Part model, mm, in its own coordinate system. A direction names the side the tool comes from. Coordinates: 2 decimals unless noted, no trailing zeros. Order: outer loops, then holes, each group sorted by start corner. A loop starts at its lowest first (then second) coordinate and runs counter-clockwise, first axis right, second up. Notation, with made-up numbers: (1.5, 36) - (10.5, 36) arc R20 ccw to (10.5, 62) - close; hole circle Ø8 at (28, 52). An arc over 180 degrees is marked (long way). Use a Markdown table: item, result. Add a question column.
1) Two-plate mould, pull along Y, no slides. Class faces 3 (the face through (1, -18, -45)), 4 (the face through (1.5, -15.9, -6.3)), 5 (the face through (1, -15, -30)): +Y half, -Y half, draft (parallel to the pull), parting line (faces both ways), or undercut.
2) Tool access for faces 1 (the face through (1, -18, -15)), 2 (the face through (1.5, -15.9, -51.3)): list every direction of +Z, -Z, +X, -X, +Y, -Y with a clear straight run to the whole face (end or side of a thin tool).
3) Wall check: L1, parallel to Y at x = 0.7, z = -7.5; L2, parallel to Y at x = 2.2, z = -17.5; L3, parallel to Z at x = 0.7, y = -18.5. Give the ranges that are in metal, low to high. Write a range as [from, to].
4) Saw through at B-B on y = -8.25. List the corners of the cut face in (x, z), then the cut area to 3 significant figures.
5) Saw through at D-D on z = -42.5. List the corners of the cut face in (x, y), then the cut area to 3 significant figures.
6) Saw through at C-C on x = 1.1. List the corners of the cut face in (y, z).
7) Saw through at A-A on z = -7.5. List the corners of the cut face in (x, y), then the cut area to 3 significant figures.
```python
from build123d import *

# Parameters (mm, degrees)
EXTRUDE_1_DEPTH     = 3
SKETCH_2_R          = 1.5
CUT_EXTRUDE_1_DEPTH = 3


with BuildPart() as part:
    # 草图1 → 凸台-拉伸1 (new body)
    with BuildSketch(Plane(origin=(0, 0, 0), x_dir=(0, 0, -1), z_dir=(1, 0, 0))):
        Polygon((0, 0), (60, 0), (60, -21), (45, -21), (45, -15), (15, -15), (15, -21), (0, -21), align=None)
    extrude(amount=EXTRUDE_1_DEPTH)

    # 草图2 → 切除-拉伸1 (cut)
    with BuildSketch(Plane(origin=(3, 0, 0), x_dir=(0, 0, -1), z_dir=(1, 0, 0))):
        with Locations((42.5, -7.5)):
            Circle(SKETCH_2_R)
        with Locations((17.5, -7.5)):
            Circle(SKETCH_2_R)
        with Locations((52.5, -15)):
            Circle(SKETCH_2_R)
        with Locations((7.5, -15)):
            Circle(SKETCH_2_R)
    extrude(amount=-CUT_EXTRUDE_1_DEPTH, mode=Mode.SUBTRACT)


solid = part.part
```
Results are:
| question | item | result |
|---|---|---|
| 1 | face 3 | draft |
| 1 | face 4 | undercut |
| 1 | face 5 | -Y half |
| 2 | face 1 | +X, -X, -Y |
| 2 | face 2 | +X, -X |
| 3 | L1 | [-21, -16.5], [-13.5, 0] |
| 3 | L2 | [-15, -9], [-6, 0] |
| 3 | L3 | [-60, -45], [-15, 0] |
| 4 | outline | (0, -60) - (3, -60) - (3, -43.8) - (0, -43.8) - close; (0, -41.2) - (3, -41.2) - (3, -18.8) - (0, -18.8) - close; (0, -16.2) - (3, -16.2) - (3, 0) - (0, 0) - close |
| 4 | area | 164 mm2 |
| 5 | outline | (0, -15) - (3, -15) - (3, -9) - (0, -9) - close; (0, -6) - (3, -6) - (3, 0) - (0, 0) - close |
| 5 | area | 36.0 mm2 |
| 6 | outline | (-21, -60) - (0, -60) - (0, 0) - (-21, 0) - (-21, -15) - (-15, -15) - (-15, -45) - (-21, -45) - close; hole circle Ø3 at (-15, -52.5); hole circle Ø3 at (-15, -7.5); hole circle Ø3 at (-7.5, -42.5); hole circle Ø3 at (-7.5, -17.5) |
| 7 | outline | (0, -21) - (3, -21) - (3, -16.5) - (0, -16.5) - close; (0, -13.5) - (3, -13.5) - (3, 0) - (0, 0) - close |
| 7 | area | 54.0 mm2 |
